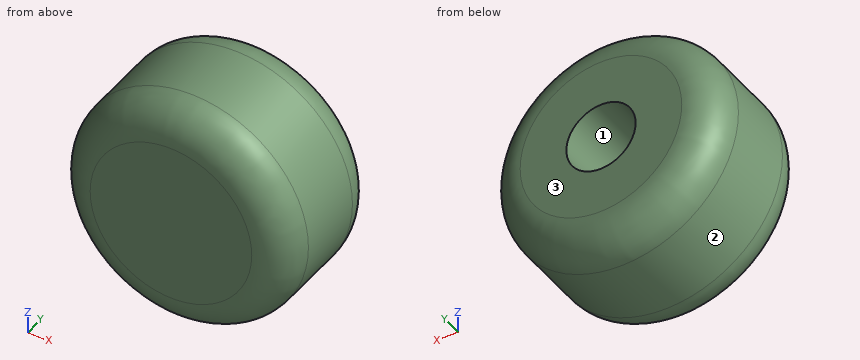
```python
from build123d import *

# Parameters (mm, degrees)
F0_R     = 10
F1_DEPTH = 12
F2_R     = 3
F4_D     = 6
F4_DEPTH = 8
F4_TIP   = 1.8025818571


with BuildPart() as f1:
    # F0 (on Front) → F1 (new body)
    with BuildSketch(Plane.XZ):
        Circle(F0_R)
    extrude(amount=F1_DEPTH)

    # F2
    f2_edges = [f1.edges().sort_by_distance(p)[0] for p in [
        (-10, 0, 0),
        (-10, -12, 0),
    ]]
    fillet(f2_edges, radius=F2_R)

    # F4
    with Locations(Plane(origin=(0, 0, 0), x_dir=(1, 0, 0), z_dir=(0, 1, 0))):
        with Locations((0, 0)):
            Hole(F4_D / 2, depth=F4_DEPTH)
            with Locations((0, 0, -(F4_DEPTH + F4_TIP / 2))):  # 118° drill point
                Cone(0, F4_D / 2, F4_TIP, mode=Mode.SUBTRACT)


solid = f1.part
```
Work out the finished part from the listing and answer in its coordinate system (mm). Face numbers are marked on the shaded views. Coordinates: 2 decimals unless noted, no trailing zeros. Write each loop counter-clockwise with the first axis right and the second up, starting at its lowest first coordinate (ties: lowest second). Pieces come first, ordered by that corner, then holes. Notation, with made-up numbers: (46.25, -32.75) - (66.25, -32.75) arc R28 cw to (66.25, -11.75) - close; hole circle Ø5 at (55, -15). An arc over 180 degrees is marked (long way). Answer as a JSON object with one key per item and string values.
Q1. For a pull along X with two mould halves and no side action, classify the marked faces 1, 2 and 3 as pulls with the +X half, pulls with the -X half, needs draft (parallel to the pull), parting line crosses it, or undercut.
Results list:
{"face 1": "undercut", "face 2": "parting line crosses it", "face 3": "needs draft"}
Q2. Find section B-B (y = -11). Write down the section's boundary in (x, z).
Results list:
{"outline": "circle Ø18.47 at (0, 0)"}
Q3. Given pin 1 Ø1.5 at (x, z) = (-7, -7) entering from +Y; pin 2 Ø4 at (x, y) = (1, -3.5) entering from -Z; pin 3 Ø5 at (x, y) = (-7, -5.5) entering from +Z, each flat-ended and moving along its own axis, determine where each tip first touches the part or whether it passes through.
Results list:
{"pin 1": "stops at y = -0.91", "pin 2": "stops at z = -10", "pin 3": "stops at z = 8.93"}
Q4. Consider L1, parallel to Z at x = 0, y = -4.75; L2, parallel to X at y = -0.75, z = 1.5; L3, parallel to Z at x = -1.5, y = -2. Determine where each line is inside the solid, lowest interval first. Write a range as from..to.
Results list:
{"L1": "z = -10..-3, 3..10", "L2": "x = -8.86..-2.6, 2.6..8.86", "L3": "z = -9.71..-2.6, 2.6..9.71"}
Q5. Find section A-A (y = -3.5). Write down the section's boundary in (x, z), plus the area to 3 significant figures.
Results list:
{"outline": "circle Ø20 at (0, 0); hole circle Ø6 at (0, 0)", "area": "286 mm^2"}
